Verification items for the finished model (mm, model axes). Round coordinates to 2 decimals unless told otherwise and drop trailing zeros. Write each loop counter-clockwise with the first axis right and the second up, starting at its lowest first coordinate (ties: lowest second). Pieces come first, ordered by that corner, then holes. Notation, with made-up numbers: (-4, 14) -> (44, 14) arc R25 cw to (44, 44) -> close; hole circle Ø9 at (-3.75, 8.25). An arc over 180 degrees is marked (long way). Answer as a JSON object with one key per item and string values. Group by question number.
(1) Sectioned sample at C-C on z = 0. Record the cut outline in (x, y).
(2) Sectioned sample at A-A on x = 0. Count the separate pieces of the cut face and the enclosed holes in it, and give its area (3 significant figures).
(3) Draft check along Y on faces 1 (the face through (0.077, 3.219, 31.623)), 2 (the face through (29, 6.35, -6)), 3 (the face through (29, 0, -6)). Enter one of: released by +Y, released by -Y, zero draft, split by the parting line, or undercut.
(4) Gauge pin test, flat ends, axial feed: pin 1 Ø3 at (x, y) = (-11, 5) entering from +Z; pin 2 Ø8 at (x, z) = (-17, -13) entering from -Y. Record the tip position at first contact, or that the pin passes through.
(5) Sectioned sample at D-D on x = 16. Record the cut outline in (y, z), and give its area (3 significant figures).
(6) Scan lines: L1, parallel to X at y = 2, z = 0; L2, parallel to X at y = 5, z = -12; L3, parallel to Z at x = 26.5, y = 4. Record each from-to range of solid material in increasing order. Write a range as from..to.
```python
from build123d import *

# Parameters (mm, degrees)
SKETCH1_R           = 38.2905
SKETCH1_R_2         = 28.702
BOSS_EXTRUDE1_DEPTH = 6.35
CUT_EXTRUDE1_DEPTH  = 6.35
FILLET1_R           = 0.889


with BuildPart() as part:
    # Sketch1 → Boss-Extrude1 (new body)
    with BuildSketch(Plane(origin=(0, 0, 0), x_dir=(1, 0, 0), z_dir=(0, 1, 0))):
        with Locations(Location((0, 0, 0), (0, 0, 270))):
            Circle(SKETCH1_R)
        with Locations(Location((0, 0, 0), (0, 0, 270))):
            Circle(SKETCH1_R_2, mode=Mode.SUBTRACT)
    extrude(amount=BOSS_EXTRUDE1_DEPTH)

    # Sketch2 → Cut-Extrude1 (cut)
    with BuildSketch(Plane(origin=(0, 6.35, 0), x_dir=(1, 0, 0), z_dir=(0, 1, 0))):
        with BuildLine():
            ThreePointArc((6.3246, 30.984085654), (0, 31.623), (-6.3246, 30.984085654))
            Line((-6.3246, 30.984085654), (-6.985, 34.219371707))
            ThreePointArc((-6.985, 34.219371707), (0, 34.925), (6.985, 34.219371707))
            Line((6.985, 34.219371707), (6.3246, 30.984085654))
        make_face()
        with BuildLine():
            ThreePointArc((6.3246, -30.984085654), (0, -31.623), (-6.3246, -30.984085654))
            Line((-6.3246, -30.984085654), (-6.985, -34.219371707))
            ThreePointArc((-6.985, -34.219371707), (0, -34.925), (6.985, -34.219371707))
            Line((6.985, -34.219371707), (6.3246, -30.984085654))
        make_face()
    extrude(amount=-CUT_EXTRUDE1_DEPTH, mode=Mode.SUBTRACT)

    # Fillet1
    fillet1_edges = [part.edges().sort_by_distance(p)[0] for p in [
        (6.3246, 3.175, -30.984085654),
        (-6.3246, 3.175, -30.984085654),
        (-6.985, 3.175, -34.219371707),
        (6.985, 3.175, -34.219371707),
        (-6.985, 3.175, 34.219371707),
        (-6.3246, 3.175, 30.984085654),
        (6.3246, 3.175, 30.984085654),
        (6.985, 3.175, 34.219371707),
    ]]
    fillet(fillet1_edges, radius=FILLET1_R)


solid = part.part
```
Computed values:
{
 "1": {"outline": "(-38.29, 0) -> (-28.7, 0) -> (-28.7, 6.35) -> (-38.29, 6.35) -> close; (28.7, 0) -> (38.29, 0) -> (38.29, 6.35) -> (28.7, 6.35) -> close"},
 "2": {"separate pieces": "4", "enclosed holes": "0", "area": "79.8 mm2"},
 "3": {"face 1": "zero draft", "face 2": "released by +Y", "face 3": "released by -Y"},
 "4": {"pin 1": "z = 37.09", "pin 2": "through"},
 "5": {"outline": "(0, -34.79) -> (6.35, -34.79) -> (6.35, -23.83) -> (0, -23.83) -> close; (0, 23.83) -> (6.35, 23.83) -> (6.35, 34.79) -> (0, 34.79) -> close", "area": "139 mm2"},
 "6": {"L1": "-38.29..-28.7, 28.7..38.29", "L2": "-36.36..-26.07, 26.07..36.36", "L3": "-27.64..-11.03, 11.03..27.64"}
}
